```python
from build123d import *

# Parameters (mm, degrees)
SKETCH1_R                                      = 8.89
BOSS_EXTRUDE1_DEPTH                            = 12.7
CUT_EXTRUDE2_START                             = -10.16
CUT_EXTRUDE2_DEPTH                             = 6.35
CSK_FOR_8_FLAT_HEAD_MACHINE_SCREW1_D           = 4.4958
CSK_FOR_8_FLAT_HEAD_MACHINE_SCREW1_CSINK_D     = 8.4328
CSK_FOR_8_FLAT_HEAD_MACHINE_SCREW1_CSINK_ANGLE = 82
FILLET1_R                                      = 25.4


with BuildPart() as part:
    # Sketch1 → Boss-Extrude1 (new body)
    with BuildSketch(Plane(origin=(0, 0, 0), x_dir=(1, 0, 0), z_dir=(0, 1, 0))):
        Circle(SKETCH1_R)
        with BuildLine():
            Line((0, -25.992621117), (8.353867399, -3.040559074))
            ThreePointArc((8.353867399, -3.040559074), (0, -8.89), (-8.353867399, -3.040559074))
            Line((-8.353867399, -3.040559074), (0, -25.992621117))
        make_face()
    extrude(amount=BOSS_EXTRUDE1_DEPTH)

    # Sketch5 → Cut-Extrude2 (cut)
    with BuildSketch(Plane(origin=(0, 12.7, 0), x_dir=(1, 0, 0), z_dir=(0, 1, 0)).offset(CUT_EXTRUDE2_START)):
        with BuildLine():
            Line((-4.445, 0), (-4.445, 0.512896595))
            ThreePointArc((-4.445, 0.512896595), (-2.977090499, 3.340362268), (0, 4.474493035))
            Line((0, 4.474493035), (0, 8.89))
            ThreePointArc((0, 8.89), (-7.282261674, 5.099094519), (-8.353867399, -3.040559074))
            Line((-8.353867399, -3.040559074), (0, -25.992621117))
            Line((0, -25.992621117), (-4.445, 0))
        make_face()
    cut_extrude2 = extrude(amount=CUT_EXTRUDE2_DEPTH, mode=Mode.SUBTRACT)

    # CSK for #8 Flat Head Machine Screw1 (through all)
    with Locations(Plane(origin=(0, 12.7, 0), x_dir=(1, 0, 0), z_dir=(0, 1, 0))):
        with Locations((0, 0)):
            CounterSinkHole(CSK_FOR_8_FLAT_HEAD_MACHINE_SCREW1_D / 2, CSK_FOR_8_FLAT_HEAD_MACHINE_SCREW1_CSINK_D / 2, counter_sink_angle=CSK_FOR_8_FLAT_HEAD_MACHINE_SCREW1_CSINK_ANGLE)

    # Mirror1: Cut-Extrude2 across plane
    add(cut_extrude2.mirror(Plane(origin=(0, 0, 0), x_dir=(0, 0, 1), z_dir=(1, 0, 0))), mode=Mode.SUBTRACT)

    # Fillet1
    # the kernel refuses this fillet: 25.4 mm, written as the material it takes off along each edge
    with BuildSketch(Plane(origin=(-4.445, 2.54, 0), x_dir=(0, 0, -1), z_dir=(0, 1, 0))) as fillet1_piece_1:
        with BuildLine():
            CenterArc((2.715876885, -25.30428576), FILLET1_R, 94.975600716, 4.728682493)
            Line((-1.565625003, -0.267737644), (-1.65125504, 0.232993318))
            Line((-1.65125504, 0.232993318), (-0.085630038, 0.500730962))
            Line((-0.085630038, 0.500730962), (0, 0.508))
            ThreePointArc((0, 0.508), (0.256448297, 0.508), (0.468836989, 0.506085715))
            Line((0.468836989, 0.506085715), (0.512896595, 0))
        make_face()
    extrude(amount=6.35, mode=Mode.SUBTRACT)
    with BuildSketch(Plane(origin=(4.445, 2.54, 0), x_dir=(-0.16856306644022723, 0, 0.9856908707258414), z_dir=(0, 1, 0))) as fillet1_piece_2:
        with BuildLine():
            CenterArc((1.58835295, -25.4), FILLET1_R, 90, 4.728682493)
            Line((-0.505557491, -0.086455423), (-0.5474357, 0.419815469))
            ThreePointArc((-0.5474357, 0.419815469), (-0.338408783, 0.457503251), (-0.085630038, 0.500730962))
            Line((-0.085630038, 0.500730962), (0, 0.508))
            Line((0, 0.508), (1.58835295, 0.508))
            Line((1.58835295, 0.508), (1.58835295, 0))
        make_face()
    extrude(amount=6.35, mode=Mode.SUBTRACT)


solid = part.part
```
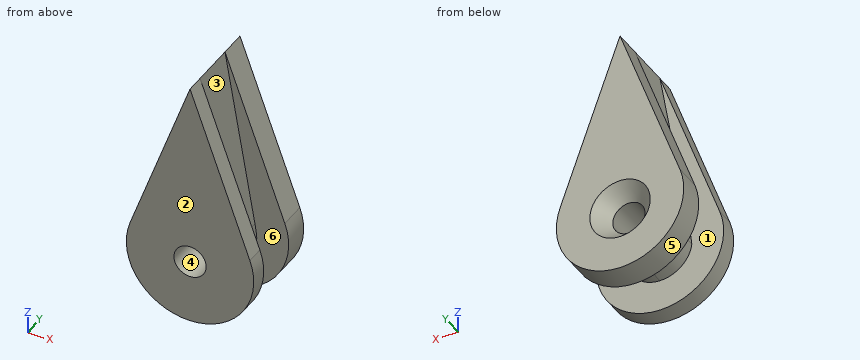
CAD build for the part. Positions are in the model's coordinates, mm. Face numbers are marked on the shaded views. A direction names the side the tool comes from. Give positions to 0.01 mm unless a question says otherwise; leave off trailing zeros. Loops run counter-clockwise (first coordinate to the right, second up) from the corner with the lowest first, then second, coordinate; pieces in that order, holes last. Notation, with made-up numbers: (38.25, 58) - (48.25, 58) arc R23 cw to (48.25, 72) - close; hole circle Ø11 at (27.5, 14). An arc over 180 degrees is marked (long way). Put each result on its own line as item: value.
Q1. Slice it at C-C (x = 5.5). Give the cut face in (y, z), plus the area to 3 significant figures.
Filled in:
outline: (0, -6.98) - (2.54, -6.98) - (2.54, 10.88) - (0, 10.88) - close; (8.89, -6.98) - (12.7, -6.98) - (12.7, 10.88) - (8.89, 10.88) - close
area: 113 mm²
Q2. Mould opens along Z. For the marked faces 4, 5 and 6 say: pulls with the +Z half, pulls with the -Z half, needs draft (parallel to the pull), parting line crosses it, or undercut.
Filled in:
face 4: undercut
face 5: parting line crosses it
face 6: needs draft
Q3. Slice it at D-D (z = 23). Give the cut face in (x, y).
Filled in:
outline: (-1.09, 0) - (1.09, 0) - (1.09, 2.54) - (0.51, 2.54) - (0.51, 8.89) - (1.09, 8.89) - (1.09, 12.7) - (-1.09, 12.7) - (-1.09, 8.89) - (-0.51, 8.89) - (-0.51, 2.54) - (-1.09, 2.54) - close
Q4. Slice it at B-B (z = 0). Give the cut face in (x, y).
Filled in:
outline: (-8.89, 0) - (-2.25, 0) - (-2.25, 10.44) - (-4.22, 12.7) - (-8.89, 12.7) - (-8.89, 8.89) - (-4.4, 8.89) - (-4.4, 2.54) - (-8.89, 2.54) - close; (2.25, 0) - (8.89, 0) - (8.89, 2.54) - (4.4, 2.54) - (4.4, 8.89) - (8.89, 8.89) - (8.89, 12.7) - (4.22, 12.7) - (2.25, 10.44) - close
Q5. Flat gauge pins, fed straight in: pin 1 (4 mm diameter, centred on y = 1.5, z = 10.5, fed in from -X); pin 2 (5 mm diameter, centred on y = 11, z = -5.5, fed in from +X); pin 3 (6 mm diameter, centred on x = 0, z = 0, fed in from +Y). Where does each tip first touch, or does it go through?
Filled in:
pin 1: stops at x = -6.37
pin 2: stops at x = 8.37
pin 3: stops at y = 11.3
Q6. Probe line 1 along Y through (x, z) = (-3.25, -7); line 2 along X through (y, z) = (4.5, -2); line 3 along X through (y, z) = (2.25, 1). List the from-to ranges inside material, lowest first.
Filled in:
line 1: y = 0 to 2.54, 8.89 to 12.7
line 2: x = -4 to -1.03, 1.03 to 4
line 3: x = -8.83 to -2.01, 2.01 to 8.83
Q7. Tool access for the marked faces 1, 2 and 3: list every direction of +Z, -Z, +X, -X, +Y, -Y with a clear straight run to the whole face (end or side of a thin tool).
Filled in:
face 1: none
face 2: +Z, -Z, +X, -X, -Y
face 3: +Z, +X
Q8. Slice it at A-A (y = 8.5). Give the cut face in (x, z) (1 decimal).
Filled in:
outline: (-4.4, -0.5) arc R4.5 ccw to (4.4, -0.5) arc R25.4 ccw to (4.2, 1.6) - (0, 26) - (-4.2, 1.6) arc R25.4 ccw to start; hole circle Ø4.5 at (0, 0)
